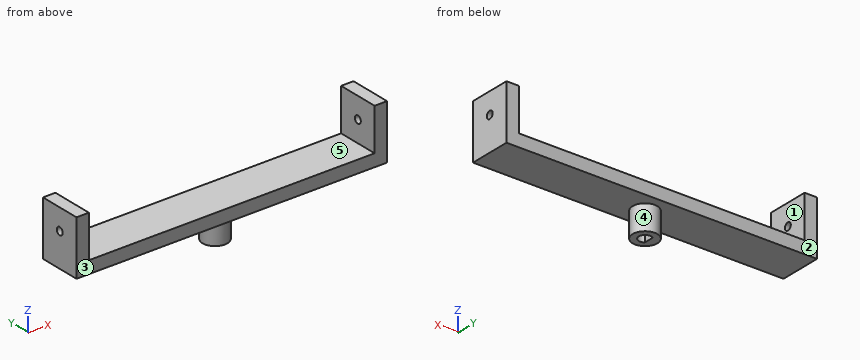
Autodesk Inventor part; units mm, degrees
ref_plane "YZ Plane" through (0, 0, 0) normal (1, 0, 0) x (0, 1, 0)
ref_plane "XZ Plane" through (0, 0, 0) normal (0, 1, 0) x (-1, 0, 0)
ref_plane "XY Plane" through (0, 0, 0) normal (0, 0, 1) x (1, 0, 0)
sketch "Sketch1" plane through (0, 0, 0) normal (0, 0, 1) x (1, 0, 0)
  circle A0 centre (0, 0) radius 5
  arc A1 (-1.5, -2) -> (-1.5, 2) centre (0, 0) ccw
  line L0 (-1.5, 2) -> (-1.5, -2)
  dimension "d0" = 10
extrude "Extrusion1" add sketch "Sketch1" against normal blind 10
sketch "Sketch2" plane through (0, 0, 0) normal (0, 0, 1) x (1, 0, 0)
  line L0 (-17.5, 8.5) -> (17.5, 8.5)
  line L1 (17.5, 8.5) -> (17.5, -8.5)
  line L2 (17.5, -8.5) -> (-17.5, -8.5)
  line L3 (-17.5, -8.5) -> (-17.5, 8.5)
  line L4 (-17.5, 8.5) -> (17.5, -8.5) construction
  line L5 (17.5, 8.5) -> (-17.5, -8.5) construction
  point P0 (0, 0)
  dimension "d3" = 35
  dimension "d4" = 17
extrude "Extrusion2" add sketch "Sketch2" along normal blind 5
sketch "Sketch3" plane through (-17.5, -8.5, 0) normal (-1, 0, 0) x (0, 0, 1)
  line L0 (0, 0) -> (5, 0)
  line L1 (5, 0) -> (5, 17)
  line L2 (0, 0) -> (5, 0)
  line L3 (5, 0) -> (5, 17)
  line L4 (5, 17) -> (0, 17)
  line L5 (0, 17) -> (0, 0)
  point P0 (0, 8.5)
extrude "Extrusion3" add sketch "Sketch3" along normal blind 45
sketch "Sketch4" plane through (17.5, -8.5, 0) normal (1, 0, 0) x (0, 0, -1)
  line L0 (0, 0) -> (0, 17)
  line L1 (-5, 0) -> (-5, 17)
  line L2 (0, 0) -> (-5, 0)
  line L3 (-5, 0) -> (-5, 17)
  line L4 (-5, 17) -> (0, 17)
  line L5 (0, 17) -> (0, 0)
  point P0 (0, 8.5)
extrude "Extrusion4" add sketch "Sketch4" along normal blind 45
sketch "Sketch5" plane through (0, 0, 5) normal (0, 0, 1) x (1, 0, 0)
  line L0 (62.5, -8.5) -> (-62.5, -8.5)
  line L1 (62.5, -8.5) -> (57.5, -8.5)
  line L2 (57.5, -8.5) -> (57.5, 8.5)
  line L3 (57.5, 8.5) -> (62.5, 8.5)
  line L4 (62.5, 8.5) -> (62.5, -8.5)
  point P0 (0, 0)
  dimension "d11" = 5
  dimension "d12" = 17
extrude "Extrusion5" add sketch "Sketch5" along normal blind 17
sketch "Sketch6" plane through (0, 0, 5) normal (0, 0, 1) x (1, 0, 0)
  line L0 (-62.5, -8.5) -> (62.5, -8.5)
  line L1 (-62.5, 8.5) -> (-57.5, 8.5)
  line L2 (-57.5, 8.5) -> (-57.5, -8.5)
  line L3 (-57.5, -8.5) -> (-62.5, -8.5)
  line L4 (-62.5, -8.5) -> (-62.5, 8.5)
  point P0 (0, 0)
  dimension "d15" = 5
extrude "Extrusion6" add sketch "Sketch6" along normal blind 17
sketch "Sketch7" plane through (-62.5, -8.5, 0) normal (-1, 0, 0) x (0, 0, 1)
  line L0 (0, 0) -> (22, 0)
  line L1 (22, 0) -> (5, 0)
  line L2 (5, 0) -> (5, 17)
  line L3 (5, 17) -> (22, 17)
  line L4 (22, 17) -> (22, 0)
  line L5 (5, 17) -> (22, 0)
  line L6 (5, 0) -> (22, 17)
  circle A0 centre (13.5, 8.5) radius 1.5
  point P0 (0, 8.5)
  dimension "d18" = 17
  dimension "d19" = 17
  dimension "d20" = 3
extrude "Extrusion7" cut sketch "Sketch7" against normal through all contours A0 L5 L6 | L6 L5 A0 | L5 L6 A0 | A0 L6 L5
properties part number "z axis base"
For this review, take the finished solid that the model builds, in its own axes (mm). Face numbers are marked on the shaded views. A direction names the side the tool comes from. Coordinates: 2 decimals unless noted, no trailing zeros. Order: outer loops, then holes, each group sorted by start corner. A loop starts at its lowest first (then second) coordinate and runs counter-clockwise, first axis right, second up. Notation, with made-up numbers: (7.5, 62.25) - (17.5, 62.25) arc R23 cw to (17.5, 80.25) - close; hole circle Ø6 at (7.5, 41.25). An arc over 180 degrees is marked (long way). Answer as a JSON object with one key per item and string values. Group by question number.
1. We need section C-C on x = 0. State the section outline as (y, z) points, then the cut area to 3 significant figures.
2. For probe 1 along X at (y, z) = (-7, 5.5); probe 2 along Z at (x, y) = (-60.9, 0); probe 3 along Y at (x, z) = (59.85, 13.5), list the stretches that pass through material, from the lowest coordinate up.
3. Clearance check with flat-ended pins moving along their axes: P1, Ø8, axis at x = 0, y = 0, coming from the -Z side; P2, Ø2, axis at x = 1, y = -0.5, coming from the -Z side; P3, Ø1.5, axis at x = 25.5, y = -4.5, coming from the +Z side; P4, Ø2, axis at y = -0.5, z = -3, coming from the +X side. State where each tip first meets the part, or that it passes through.
4. For the marked faces 1 and 2, list the 3-axis set-ups (+Z, -Z, +X, -X, +Y, -Y) from which the entire face can be reached by the end or side of a thin tool; tool diameter is ignored.
5. The part is to be moulded in two halves that separate along X. For the marked faces 3, 4 and 5, say which applies: pulls with the +X half, pulls with the -X half, needs draft (parallel to the pull), parting line crosses it, or undercut.
6. We need section B-B on y = 0. State the section outline as (x, z) points, then the cut area to 3 significant figures.
7. We need section D-D on y = -7. State the section outline as (x, z) points, then the cut area to 3 significant figures.
8. We need section A-A on z = 17. State the section outline as (x, y) points.
Final values:
{
 "1": {"outline": "(-8.5, 0) - (-5, 0) - (-5, -10) - (-2.5, -10) - (-2.5, 0) - (2.5, 0) - (2.5, -10) - (5, -10) - (5, 0) - (8.5, 0) - (8.5, 5) - (-8.5, 5) - close", "area": "135 mm²"},
 "2": {"probe 1": "-62.5 to -57.5, 57.5 to 62.5", "probe 2": "0 to 12, 15 to 22", "probe 3": "-8.5 to -1.5, 1.5 to 8.5"},
 "3": {"P1": "z = -10", "P2": "z = 0", "P3": "z = 5", "P4": "x = 5"},
 "4": {"face 1": "+Z, +Y, -Y", "face 2": "+Z, -Z, +X, -X, +Y"},
 "5": {"face 3": "needs draft", "face 4": "parting line crosses it", "face 5": "undercut"},
 "6": {"outline": "(-62.5, 0) - (-5, 0) - (-5, -10) - (-1.5, -10) - (-1.5, 0) - (2.5, 0) - (2.5, -10) - (5, -10) - (5, 0) - (62.5, 0) - (62.5, 12) - (57.5, 12) - (57.5, 5) - (-57.5, 5) - (-57.5, 12) - (-62.5, 12) - close; (-62.5, 15) - (-57.5, 15) - (-57.5, 22) - (-62.5, 22) - close; (57.5, 15) - (62.5, 15) - (62.5, 22) - (57.5, 22) - close", "area": "825 mm²"},
 "7": {"outline": "(-62.5, 0) - (62.5, 0) - (62.5, 22) - (57.5, 22) - (57.5, 5) - (-57.5, 5) - (-57.5, 22) - (-62.5, 22) - close", "area": "795 mm²"},
 "8": {"outline": "(-62.5, -8.5) - (-57.5, -8.5) - (-57.5, 8.5) - (-62.5, 8.5) - close; (57.5, -8.5) - (62.5, -8.5) - (62.5, 8.5) - (57.5, 8.5) - close"}
}
